from build123d import *

# Parameters (mm, degrees)
SALIENTE_EXTRUIR1_DEPTH = 9.9
CORTAR_EXTRUIR1_DEPTH   = 8
CROQUIS3_R              = 2.5
SALIENTE_EXTRUIR2_DEPTH = 15
CROQUIS4_R              = 1.45
CORTAR_EXTRUIR2_DEPTH   = 14
CHAFL_N1_SIZE           = 0.5
CHAFL_N2_SIZE           = 0.5


with BuildPart() as part:
    # Croquis1 → Saliente-Extruir1 (new body)
    with BuildSketch(Plane.XY):
        Polygon((4.58993464, 0), (2.29496732, 3.975), (-2.29496732, 3.975), (-4.58993464, 0), (-2.29496732, -3.975), (2.29496732, -3.975), align=None)
    extrude(amount=SALIENTE_EXTRUIR1_DEPTH)

    # Croquis2 → Cortar-Extruir1 (cut)
    with BuildSketch(Plane.XY.offset(9.9)):
        with BuildLine():
            Line((-1.336974196, 1.05), (1.336974196, 1.05))
            ThreePointArc((1.336974196, 1.05), (0, -1.7), (-1.336974196, 1.05))
        make_face()
    extrude(amount=-CORTAR_EXTRUIR1_DEPTH, mode=Mode.SUBTRACT)

    # Croquis3 → Saliente-Extruir2 (add)
    with BuildSketch(Plane(origin=(0, 0, 0), x_dir=(-1, 0, 0), z_dir=(0, 0, -1))):
        Circle(CROQUIS3_R)
    extrude(amount=SALIENTE_EXTRUIR2_DEPTH)

    # Croquis4 → Cortar-Extruir2 (cut)
    with BuildSketch(Plane(origin=(0, 0, -15), x_dir=(-1, 0, 0), z_dir=(0, 0, -1))):
        Circle(CROQUIS4_R)
    extrude(amount=-CORTAR_EXTRUIR2_DEPTH, mode=Mode.SUBTRACT)

    # Chaflán1
    chafl_n1_edges = [part.edges().sort_by_distance(p)[0] for p in [
        (0, -3.975, 0),
        (-3.44245098, -1.9875, 0),
        (-3.44245098, 1.9875, 0),
        (0, 3.975, 0),
        (3.44245098, 1.9875, 0),
        (3.44245098, -1.9875, 0),
    ]]
    chamfer(chafl_n1_edges, length=CHAFL_N1_SIZE)

    # Chaflán2
    chafl_n2_edges = [part.edges().sort_by_distance(p)[0] for p in [
        (1.45, 0, -15),
    ]]
    chamfer(chafl_n2_edges, length=CHAFL_N2_SIZE)


solid = part.part
Source: CAD feature listing. Evaluate the final solid. Frame: model axes, mm. A direction names the side the tool comes from. Coordinates: 2 decimals unless noted, no trailing zeros. Loops run counter-clockwise (first coordinate to the right, second up) from the corner with the lowest first, then second, coordinate; pieces in that order, holes last. Notation, with made-up numbers: M 81,-24 L 110,-24 A29 ccw 110,-3 Z; hole C 70,85 d2. An arc over 180 degrees is marked long. Answer in a Markdown table with one row per item.
Q1. Section A-A on x = 0. Return the cut outline in (y, z) (3 decimals), plus the area to 3 significant figures.
Answers below:
| item | result |
|---|---|
| outline | M -3.975,0.5 L -3.475,0 L -2.5,0 L -2.5,-15 L -1.95,-15 L -1.45,-14.5 L -1.45,-1 L 1.45,-1 L 1.45,-14.5 L 1.95,-15 L 2.5,-15 L 2.5,0 L 3.475,0 L 3.975,0.5 L 3.975,9.9 L 1.05,9.9 L 1.05,1.9 L -1.7,1.9 L -1.7,9.9 L -3.975,9.9 Z |
| area | 90.6 mm^2 |
Q2. Section C-C on y = -2.75. Return the cut outline in (x, z), plus the area to 3 significant figures.
Answers below:
| item | result |
|---|---|
| outline | M -3,0.5 L -2.42,0 L 2.42,0 L 3,0.5 L 3,9.9 L -3,9.9 Z |
| area | 59.2 mm^2 |
Q3. First-contact query: pin 1 (3.5 mm diameter, centred on x = 0, y = 0, fed in from -Z). Flat tip, straight axial feed; report the tip coordinate or a pass-through.
Answers below:
| item | result |
|---|---|
| pin 1 | stops at z = -14.8 |
Q4. Section B-B on z = -7.5. Return the cut outline in (x, y), plus the area to 3 significant figures.
Answers below:
| item | result |
|---|---|
| outline | C 0,0 d5; hole C 0,0 d2.9 |
| area | 13.0 mm^2 |
Q5. Section D-D on x = -3.5. Return the cut outline in (y, z), plus the area to 3 significant figures.
Answers below:
| item | result |
|---|---|
| outline | M -1.89,0.5 L -0.89,0 L 0.89,0 L 1.89,0.5 L 1.89,9.9 L -1.89,9.9 Z |
| area | 36.9 mm^2 |
Q6. Draft query along Y for faces 4 (the flat face through (0, 1.05, 6)), 5 (the flat face through (-3.245, -1.836, 0.253)), 6 (the flat face through (-3.426, 2.015, 5.134)). Return one class per face: pulls with the +Y half, pulls with the -Y half, needs draft (parallel to the pull), parting line crosses it, or undercut.
Answers below:
| item | result |
|---|---|
| face 4 | undercut |
| face 5 | pulls with the -Y half |
| face 6 | pulls with the +Y half |
Q7. Ray query, probe 1 along Y at (x, z) = (0, -10.75); probe 2 along X at (y, z) = (1, -13); probe 3 along Z at (x, y) = (-1, 0.75). Return the intervals inside material, ascending. Write a range as from..to.
Answers below:
| item | result |
|---|---|
| probe 1 | y = -2.5..-1.45, 1.45..2.5 |
| probe 2 | x = -2.29..-1.05, 1.05..2.29 |
| probe 3 | z = -1..1.9 |
Q8. Set-up query: faces 1 (the flat face through (0, -3.975, 5)), 2 (the flat face through (0, 0, 1.9)), 3 (the cylindrical face through (1.45, 0.06, -7.84)). Return all of +Z, -Z, +X, -X, +Y, -Y with unobstructed straight access to the full face (end or side cutting, diameter ignored); none if empty.
Answers below:
| item | result |
|---|---|
| face 1 | +Z, -Z, +X, -X, -Y |
| face 2 | +Z |
| face 3 | -Z |
